Verification items for the finished model (mm, model axes). Face numbers are marked on the shaded views. A direction names the side the tool comes from. Round coordinates to 2 decimals unless told otherwise and drop trailing zeros. Loops run counter-clockwise (first coordinate to the right, second up) from the corner with the lowest first, then second, coordinate; pieces in that order, holes last. Notation, with made-up numbers: (52, 30.25) - (104, 30.25) arc R17 ccw to (104, 43.25) - close; hole circle Ø1 at (-6.5, -16.75). An arc over 180 degrees is marked (long way). Use a Markdown table: item, result. Add a question column.
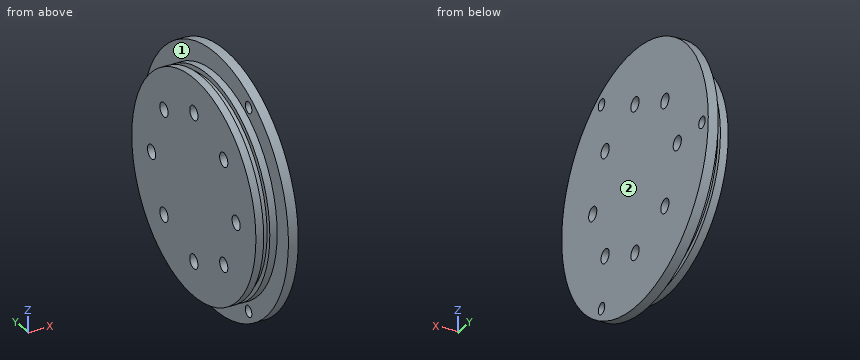
```python
from build123d import *

# Parameters (mm, degrees)
SKETCH2_R          = 4
CUT_EXTRUDE1_DEPTH = 10
CIRPATTERN1_COUNT  = 3
SKETCH3_R          = 5
CUT_EXTRUDE2_DEPTH = 23
CIRPATTERN2_COUNT  = 8


with BuildPart() as part:
    # Sketch1 → Revolve1 (revolve)
    with BuildSketch(Plane.XY):
        Polygon((0, 0), (0, 76.2), (5.475419526, 76.2), (5.475419526, 72.846582988), (9.822609824, 72.846582988), (9.822609824, 76.2), (15, 76.2), (15, 90), (22, 90), (22, 0), align=None)
    revolve(axis=Axis((22, 0, 0), (-1, 0, 0)))

    # Sketch2 → Cut-Extrude1 (cut)
    with BuildSketch(Plane.ZY.offset(-15)):
        with Locations((0, 82.277326688)):
            Circle(SKETCH2_R)
    cut_extrude1 = extrude(amount=-CUT_EXTRUDE1_DEPTH, mode=Mode.SUBTRACT)

    # CirPattern1: Cut-Extrude1 ×3 about axis
    cirpattern1_axis = Axis((0, 0, 0), (1, 0, 0))
    for i in range(1, CIRPATTERN1_COUNT):
        add(cut_extrude1.rotate(cirpattern1_axis, i * 360 / CIRPATTERN1_COUNT), mode=Mode.SUBTRACT)

    # Sketch3 → Cut-Extrude2 (cut, through all)
    with BuildSketch(Plane.ZY):
        with Locations((0, 51.916670562)):
            Circle(SKETCH3_R)
    cut_extrude2 = extrude(amount=-CUT_EXTRUDE2_DEPTH, mode=Mode.SUBTRACT)

    # CirPattern2: Cut-Extrude2 ×8 about axis
    cirpattern2_axis = Axis((0, 0, 0), (1, 0, 0))
    for i in range(1, CIRPATTERN2_COUNT):
        add(cut_extrude2.rotate(cirpattern2_axis, i * 360 / CIRPATTERN2_COUNT), mode=Mode.SUBTRACT)


solid = part.part
```
Q1. Section check D-D on z = 62. Record the cut outline in (x, y).
Q2. Set-up check for the marked faces 1 and 2: record each of +Z, -Z, +X, -X, +Y, -Y from which the full face is reachable in a straight line by a thin tool's end or side.
Q3. Section check B-B on y = 0. Record the cut outline in (x, z).
Q4. Section check C-C on x = 18.25. State how many separate pieces and enclosed holes the cut face has, plus the area to 3 significant figures.
Q5. Go/stop test with flat-tipped pins: pin 1 Ø11.5 at (y, z) = (51.92, 0) entering from +X; pin 2 Ø12 at (x, y) = (8, -65.5) entering from +Z; pin 3 Ø9 at (y, z) = (0, 51.92) entering from -X; pin 4 Ø4 at (x, z) = (6, 39.5) entering from +Y. Record where each tip stops, or that it passes through.
Q6. Section check A-A on z = 0. Record the cut outline in (x, y).
Q7. Thickness scan on line 1 along Y through (x, z) = (20, 0.5); line 2 along X through (y, z) = (-25.5, 71.5); line 3 along Y through (x, z) = (20.5, 39.5). Record the ranges inside material, lowest first.
Determined:
| question | item | result |
|---|---|---|
| 1 | outline | (0, -44.3) - (5.48, -44.3) - (5.48, -38.24) - (9.82, -38.24) - (9.82, -44.3) - (15, -44.3) - (15, -65.24) - (22, -65.24) - (22, 65.24) - (15, 65.24) - (15, 44.3) - (9.82, 44.3) - (9.82, 38.24) - (5.48, 38.24) - (5.48, 44.3) - (0, 44.3) - close |
| 2 | face 1 | -X |
| 2 | face 2 | +Z, -Z, +X, +Y, -Y |
| 3 | outline | (0, -76.2) - (5.48, -76.2) - (5.48, -72.85) - (9.82, -72.85) - (9.82, -76.2) - (15, -76.2) - (15, -90) - (22, -90) - (22, -56.92) - (0, -56.92) - close; (0, -46.92) - (22, -46.92) - (22, 46.92) - (0, 46.92) - close; (0, 56.92) - (22, 56.92) - (22, 90) - (15, 90) - (15, 76.2) - (9.82, 76.2) - (9.82, 72.85) - (5.48, 72.85) - (5.48, 76.2) - (0, 76.2) - close |
| 4 | separate pieces | 1 |
| 4 | enclosed holes | 11 |
| 4 | area | 24,700 mm² |
| 5 | pin 1 | stops at x = 22 |
| 5 | pin 2 | stops at z = 47.25 |
| 5 | pin 3 | passes through |
| 5 | pin 4 | stops at y = 66.29 |
| 6 | outline | (0, -76.2) - (5.48, -76.2) - (5.48, -72.85) - (9.82, -72.85) - (9.82, -76.2) - (15, -76.2) - (15, -90) - (22, -90) - (22, -56.92) - (0, -56.92) - close; (0, -46.92) - (22, -46.92) - (22, 46.92) - (0, 46.92) - close; (0, 56.92) - (22, 56.92) - (22, 78.28) - (15, 78.28) - (15, 76.2) - (9.82, 76.2) - (9.82, 72.85) - (5.48, 72.85) - (5.48, 76.2) - (0, 76.2) - close; (15, 86.28) - (22, 86.28) - (22, 90) - (15, 90) - close |
| 7 | line 1 | y = -90 to -56.89, -46.94 to 46.94, 56.89 to 78.31, 86.25 to 90 |
| 7 | line 2 | x = 0 to 5.48, 9.82 to 22 |
| 7 | line 3 | y = -80.87 to -40.86, -32.56 to 32.56, 40.86 to 80.87 |
